Source: three-view drawing plus pictorial views. Frame: mm from the lowest corner of the part. Give positions to 0.01 mm unless a question says otherwise; leave off trailing zeros. Loops run counter-clockwise (first coordinate to the right, second up) from the corner with the lowest first, then second, coordinate; pieces in that order, holes last. Notation, with made-up numbers: M 2,71 L 43,71 A29 cw 43,110 Z; hole C -27,-12 d9. An arc over 180 degrees is marked long. Answer as a JSON object with one key per item and string values. Group by question number.
1) Section query B-B on y = 0.35. Return loops of the section in (x, z), plus the area to 3 significant figures.
2) Section query A-A on z = 8. Return loops of the section in (x, y).
3) Ray query, L1, parallel to X at y = 0.8, z = 1.5 (1 decimal); L2, parallel to X at y = 0.3, z = 2.25 (1 decimal); L3, parallel to X at y = 0.2, z = 3.5 (1 decimal). Return the intervals inside material, ascending.
4) Section query C-C on x = 19. Return loops of the section in (y, z).
5) Section query D-D on z = 3.5. Return loops of the section in (x, y), plus the area to 3 significant figures.
6) First-contact query: P1, Ø1.8, axis at x = 21.56, z = 1.82, coming from the +Y side; P2, Ø0.6, axis at x = 27, y = 1, coming from the +Z side. Flat tips, straight axial feed; report the tip coordinate or a pass-through.
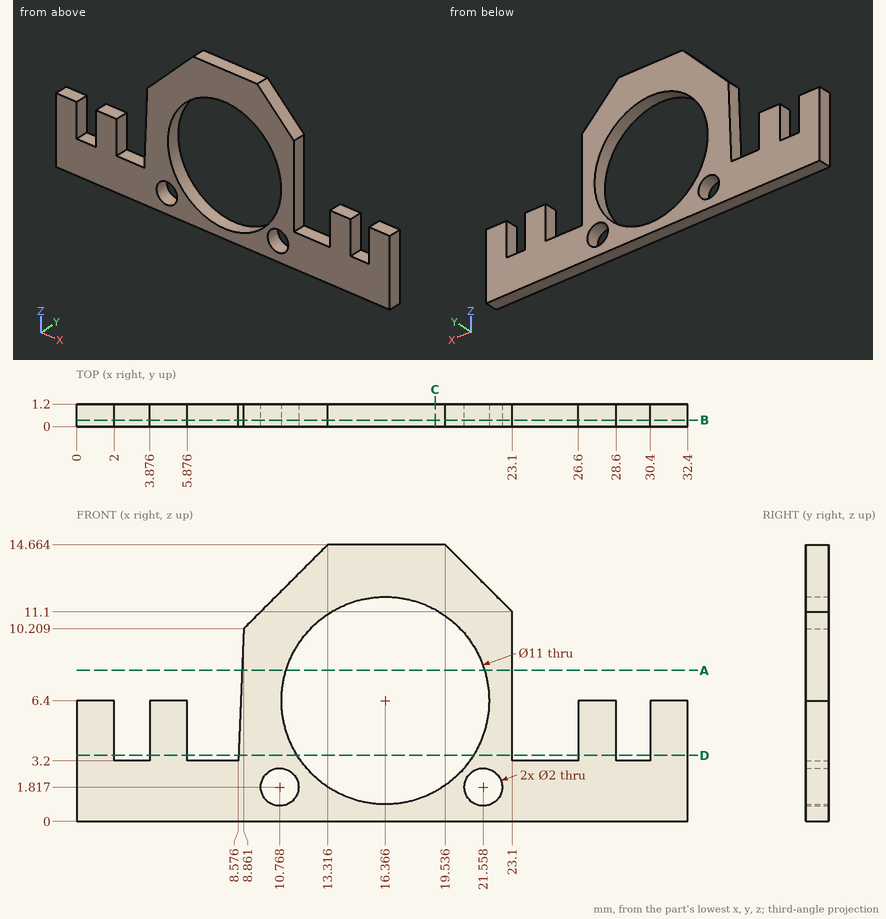
Output:
{
 "1": {"outline": "M 0,0 L 32.4,0 L 32.4,6.4 L 30.4,6.4 L 30.4,3.2 L 28.6,3.2 L 28.6,6.4 L 26.6,6.4 L 26.6,3.2 L 23.1,3.2 L 23.1,11.1 L 19.54,14.66 L 13.32,14.66 L 8.86,10.21 L 8.58,3.2 L 5.88,3.2 L 5.88,6.4 L 3.88,6.4 L 3.88,3.2 L 2,3.2 L 2,6.4 L 0,6.4 Z; hole C 10.77,1.82 d2; hole C 16.37,6.4 d11; hole C 21.56,1.82 d2", "area": "176 mm^2"},
 "2": {"outline": "M 8.77,0 L 11.1,0 L 11.1,1.2 L 8.77,1.2 Z; M 21.63,0 L 23.1,0 L 23.1,1.2 L 21.63,1.2 Z"},
 "3": {"L1": "x = 0 to 9.8, 11.7 to 13.9, 18.9 to 20.6, 22.5 to 32.4", "L2": "x = 0 to 9.9, 11.7 to 12.8, 20 to 20.7, 22.5 to 32.4", "L3": "x = 0 to 2, 3.9 to 5.9, 8.6 to 11.7, 21 to 23.1, 26.6 to 28.6, 30.4 to 32.4"},
 "4": {"outline": "M 0,0 L 1.2,0 L 1.2,1.57 L 0,1.57 Z; M 0,11.23 L 1.2,11.23 L 1.2,14.66 L 0,14.66 Z"},
 "5": {"outline": "M 0,0 L 2,0 L 2,1.2 L 0,1.2 Z; M 3.88,0 L 5.88,0 L 5.88,1.2 L 3.88,1.2 Z; M 8.59,0 L 11.69,0 L 11.69,1.2 L 8.59,1.2 Z; M 21.04,0 L 23.1,0 L 23.1,1.2 L 21.04,1.2 Z; M 26.6,0 L 28.6,0 L 28.6,1.2 L 26.6,1.2 Z; M 30.4,0 L 32.4,0 L 32.4,1.2 L 30.4,1.2 Z", "area": "15.8 mm^2"},
 "6": {"P1": "passes through", "P2": "stops at z = 6.4"}
}
